Work out the finished part from the listing and answer in its coordinate system (mm). Give positions to 0.01 mm unless a question says otherwise; leave off trailing zeros. Loops run counter-clockwise (first coordinate to the right, second up) from the corner with the lowest first, then second, coordinate; pieces in that order, holes last. Notation, with made-up numbers: (15, -2) - (59, -2) arc R10 ccw to (59, 8) - close; hole circle Ø7 at (-20.75, -7.75). An arc over 180 degrees is marked (long way). Use CSV: the item, a comma, the result in double quotes.
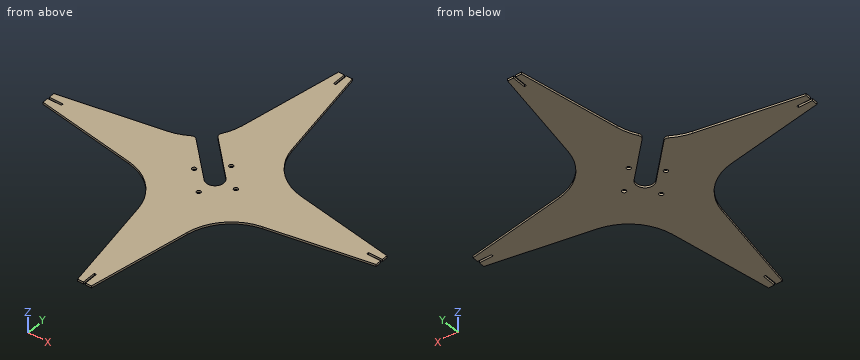
Autodesk Inventor part; units mm, degrees
ref_plane "YZ Plane" through (0, 0, 0) normal (1, 0, 0) x (0, 1, 0)
ref_plane "XZ Plane" through (0, 0, 0) normal (0, 1, 0) x (-1, 0, 0)
ref_plane "XY Plane" through (0, 0, 0) normal (0, 0, 1) x (1, 0, 0)
sketch "Sketch1" plane through (0, 0, 0) normal (0, 0, 1) x (1, 0, 0)
  circle A0 centre (0, 0) radius 37.5 construction
  circle A1 centre (0, 0) radius 12.5
  line L0 (0, 12.5) -> (35.3553, 12.5) construction
  line L1 (0, -12.5) -> (35.3553, -12.5) construction
  circle A2 centre (0, 0) radius 240
  dimension "d15" = 25
  dimension "d16" = 75
  dimension "d25" = 480
extrude "Plate1" add sketch "Sketch1" along normal blind 3
sketch "Sketch2" plane through (0, 0, 0) normal (0, 0, -1) x (-1, 0, 0)
  line L0 (18.691, -4.6928) -> (218.691, -4.6928) construction
  line L1 (218.691, -4.6928) -> (218.691, -24.6928) construction
  line L2 (218.691, -24.6928) -> (18.691, -24.6928) construction
  line L3 (18.691, -24.6928) -> (18.691, -4.6928) construction
  point P0 (0, 0)
  point P1 (-251, -525)
  dimension "d6" = 200
  dimension "d9" = 20
mark "Mark1"
sketch "Sketch4" plane through (0, 0, 3) normal (0, 0, 1) x (1, 0, 0)
  circle A0 centre (0, 0) radius 12.5 construction
  circle A1 centre (0, 0) radius 240
  line L0 (0, 0) -> (240, 0) construction
  line L1 (0, 0) -> (169.7056, 169.7056) construction
  line L2 (-10, 239.7916) -> (10, 239.7916)
  circle A2 centre (0, 0) radius 240
  line L3 (239.7916, -10) -> (239.7916, 10)
  line L4 (10, 239.7916) -> (35.3257, 96.1626)
  arc A3 (35.3257, 96.1626) -> (96.1626, 35.3257) centre (109.1862, 109.1862) ccw
  line L5 (96.1626, 35.3257) -> (239.7916, 10)
  line L6 (-1.55, 239.7916) -> (-1.55, 219.7916)
  line L7 (-1.55, 219.7916) -> (1.55, 219.7916)
  line L8 (1.55, 219.7916) -> (1.55, 239.7916)
  circle A4 centre (0, 30) radius 3
  line L9 (0, 30) -> (0, 0) construction
  circle A5 centre (0, 0) radius 30 construction
  point P0 (0, 219.7916)
  point P1 (0, 239.7916)
  point P2 (239.7916, 10)
  point P3 (10, 239.7916)
  point P4 (10, 239.7916)
  dimension "d39" = 60
  dimension "d28" = 20
  dimension "d29" = 45
  dimension "d30" = 10
  dimension "d31" = 75
  dimension "d32" = 3.1
  dimension "d33" = 20
  dimension "d40" = 90
  dimension "d41" = 6
extrude "Cut2" cut sketch "Sketch4" against normal blind 3 contours L5 A3 L4 A1 | L2 A1 | L8 L7 L6 L2 | A4
pattern_circular "Circular Pattern2" count 4 over 360 about axis through (0, 0, 0) along (0, 0, 1) of "Cut2"
sketch "Sketch5" plane through (0, 0, 3) normal (0, 0, 1) x (1, 0, 0)
  circle A0 centre (0, 0) radius 12.5
  line L0 (8.8388, 8.8388) -> (-61.8718, 79.5495)
  line L1 (-8.8388, -8.8388) -> (-79.5495, 61.8718)
  line L2 (-79.5495, 61.8718) -> (-61.8718, 79.5495)
  line L3 (0, 0) -> (0, 35.5933) construction
  dimension "d42" = 45
  dimension "d43" = 100
extrude "Cut3" cut sketch "Sketch5" against normal blind 3 contours A0 L1 L2 L0
fillet "Corner Round1" radius 6 2 edges at (-48.0562, 65.7338, 1.5) (-65.7338, 48.0562, 1.5)
equation "\"d2\" = Thickness"
equation "\"BendReliefWidth\" = Thickness"
equation "\"BendReliefDepth\" = 0.5 * Thickness"
equation "\"CornerReliefSize\" = 4 * Thickness"
equation "\"MinimumRemnant\" = 2 * Thickness"
equation "\"TransitionRadius\" = BendRadius"
equation "\"JacobiRadiusSize\" = BendRadius"
equation "\"GapSize\" = Thickness"
properties part number "TRM 030 star main" material "AISI 304"
Item 1: A cutting plane is placed at A-A on z = 0.85. State how many separate pieces and enclosed holes the cut face has, and give its area (3 significant figures).
Determined:
separate pieces,"1"
enclosed holes,"4"
area,"49,800 mm²"
Item 2: Given P1, Ø1, axis at y = 73, z = 0.5, coming from the -X side; P2, Ø1.5, axis at y = 0, z = 1.5, coming from the -X side; P3, Ø1.5, axis at x = 234.5, z = 1, coming from the -Y side, each flat-ended and moving along its own axis, determine where each tip first touches the part or whether it passes through.
Determined:
P1,"stops at x = -43.77"
P2,"stops at x = -219.79"
P3,"stops at y = -11.07"
Item 3: Find the intervals of material crossed by line 1 (Y direction, x = 0, z = 0.8); line 2 (Y direction, x = 82.5, z = 0.65); line 3 (Y direction, x = -47, z = 2.2), in increasing order.
Determined:
line 1,"y = -219.79 to -33, -27 to -12.5, 17.68 to 27, 33 to 219.79"
line 2,"y = -39.09 to 39.09"
line 3,"y = -67.26 to 29.32"
Item 4: A cutting plane is placed at B-B on y = -203.5. Determine the outline of the cut face in (x, z).
Determined:
outline,"(-16.4, 0) - (16.4, 0) - (16.4, 3) - (-16.4, 3) - close"
Item 5: A cutting plane is placed at C-C on x = 70. Determine the outline of the cut face in (y, z).
Determined:
outline,"(-45.24, 0) - (45.24, 0) - (45.24, 3) - (-45.24, 3) - close"
